```python
from build123d import *

# Parameters (mm, degrees)
BOSS_EXTRUDE1_DEPTH = 5
FILLET1_R           = 0.5


with BuildPart() as part:
    # Sketch1 → Boss-Extrude1 (new body)
    with BuildSketch(Plane.XY):
        with BuildLine():
            Line((-6, -5), (-13, -5))
            Line((-13, -5), (-13.4, -4.6))
            Line((-13.4, -4.6), (-13.4, 4))
            Line((-13.4, 4), (-13, 4.4))
            Line((-13, 4.4), (13, 4.4))
            Line((13, 4.4), (13.4, 4))
            Line((13.4, 4), (13.4, -4.6))
            Line((13.4, -4.6), (13, -5))
            Line((13, -5), (6, -5))
            Line((6, -5), (6, -3.628898526))
            ThreePointArc((6, -3.628898526), (7.67, -2.54), (6, -1.451101474))
            Line((6, -1.451101474), (6, 0))
            Line((6, 0), (-6, 0))
            Line((-6, 0), (-6, -1.451101474))
            ThreePointArc((-6, -1.451101474), (-7.67, -2.54), (-6, -3.628898526))
            Line((-6, -3.628898526), (-6, -5))
        make_face()
    extrude(amount=BOSS_EXTRUDE1_DEPTH)

    # Fillet1
    fillet1_edges = [part.edges().sort_by_distance(p)[0] for p in [
        (6, -3.628898526, 2.5),
        (6, -1.451101474, 2.5),
        (-6, -1.451101474, 2.5),
        (-6, -3.628898526, 2.5),
    ]]
    fillet(fillet1_edges, radius=FILLET1_R)


solid = part.part
```
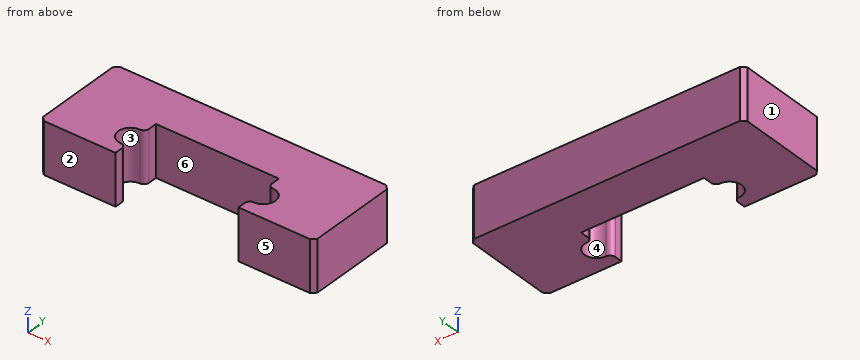
For this review, take the finished solid that the model builds, in its own axes (mm). Face numbers are marked on the shaded views. A direction names the side the tool comes from. Coordinates: 2 decimals unless noted, no trailing zeros. Order: outer loops, then holes, each group sorted by start corner. A loop starts at its lowest first (then second) coordinate and runs counter-clockwise, first axis right, second up. Notation, with made-up numbers: (5, -2.75) -> (46, -2.75) arc R34 cw to (46, 27.25) -> close; hole circle Ø4 at (-31.5, -12). An arc over 180 degrees is marked (long way). Use CSV: the item, a comma, the result in double quotes. Start each with the question number.
Item 1: Wall thickness on probe 1 along X at (y, z) = (-4.5, 0.5); probe 2 along X at (y, z) = (-2.5, 2.85); probe 3 along Y at (x, z) = (-0.25, 2.85): over which ranges is each line inside the solid? List them lowest first.
Item 2: We need section A-A, the plane y = -2.54. Give the boundary of the cut face in (x, z), then the cut area to 3 significant figures.
Item 3: For the marked faces 4, 5 and 6, list the 3-axis set-ups (+Z, -Z, +X, -X, +Y, -Y) from which the entire face can be reached by the end or side of a thin tool; tool diameter is ignored.
Item 4: Draft analysis for pull direction X (two halves, no side actions). For the marked faces 1, 2 and 3, state which applies: pulls with the +X half, pulls with the -X half, needs draft (parallel to the pull), parting line crosses it, or undercut.
Item 5: We need section B-B, the plane z = 3.2. Give the boundary of the cut face in (x, y).
Item 6: Insertion check: pin 1 (1.5 mm diameter, centred on x = -1, z = 1.5, fed in from -Y). The pin has a flat end and moves straight along its axis. Give the tip position at first contact, or say it passes through.
Derived:
1,probe 1,"x = -13.4 to -6, 6 to 13.4"
1,probe 2,"x = -13.4 to -7.67, 7.67 to 13.4"
1,probe 3,"y = 0 to 4.4"
2,outline,"(-13.4, 0) -> (-7.67, 0) -> (-7.67, 5) -> (-13.4, 5) -> close; (7.67, 0) -> (13.4, 0) -> (13.4, 5) -> (7.67, 5) -> close"
2,area,"57.3 mm^2"
3,face 4,"+Z, -Z"
3,face 5,"+Z, -Z, +X, -X, -Y"
3,face 6,"+Z, -Z, -Y"
4,face 1,"pulls with the -X half"
4,face 2,"needs draft"
4,face 3,"undercut"
5,outline,"(-13.4, -4.6) -> (-13, -5) -> (-6, -5) -> (-6, -4.23) arc R0.5 ccw to (-6.49, -3.73) arc R1.19 cw to (-6.49, -1.35) arc R0.5 ccw to (-6, -0.85) -> (-6, 0) -> (6, 0) -> (6, -0.85) arc R0.5 ccw to (6.49, -1.35) arc R1.19 cw to (6.49, -3.73) arc R0.5 ccw to (6, -4.23) -> (6, -5) -> (13, -5) -> (13.4, -4.6) -> (13.4, 4) -> (13, 4.4) -> (-13, 4.4) -> (-13.4, 4) -> close"
6,pin 1,"stops at y = 0"
